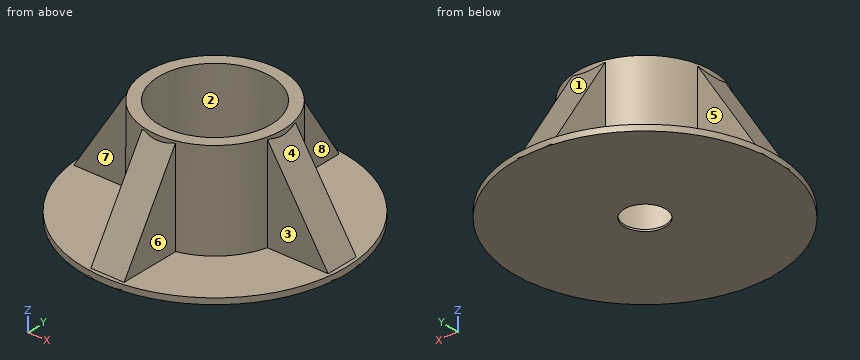
from build123d import *

# Parameters (mm, degrees)
F4_DEPTH        = 7.5
F4_COPIES_COUNT = 4


# Not quite as in the source:
# - a pattern or mirror of a feature is missing from the dataset's text; its kind, count and spacing are read off the source's solid


with BuildPart() as f2:
    # F0 (on Front) → F2 (revolve)
    with BuildSketch(Plane.XZ):
        Polygon((9.3577429652, 0), (59.3534484506, 0), (59.3534484506, 2.7155173011), (30.840517953, 2.7155173011), (30.840517953, 46.9396561384), (25.4094842821, 46.9396561384), (25.7850456983, 0.8370543364), (9.3577429652, 0.8370543364), align=None)
    revolve(axis=Axis((0, 0, 37.2192747891), (0, 0, 1)))

    # F3 (on Front) → F4 (join, symmetric)
    with BuildSketch(Plane.XZ):
        Polygon((59.184409678, 0), (30.097162351, 45.9310486913), (30.097162351, 0), align=None)
    f4 = extrude(amount=F4_DEPTH, both=True)

    # F4_copies: F4 ×4 about axis
    f4_copies_axis = Axis((0, 0, 0), (0, 0, 1))
    for i in range(1, F4_COPIES_COUNT):
        add(f4.rotate(f4_copies_axis, i * 360 / F4_COPIES_COUNT))


solid = f2.part
Verification items for the finished model (mm, model axes). Face numbers are marked on the shaded views. A direction names the side the tool comes from. Round coordinates to 2 decimals unless told otherwise and drop trailing zeros. Loops run counter-clockwise (first coordinate to the right, second up) from the corner with the lowest first, then second, coordinate; pieces in that order, holes last. Notation, with made-up numbers: (83, 69.25) - (102, 69.25) arc R21 cw to (102, 86.25) - close; hole circle Ø5 at (55, -12). An arc over 180 degrees is marked (long way). Answer in a Markdown table with one row per item. Add a question column.
Q1. Section check B-B on x = -43. Enter the section's corners in (y, z), plus the area to 3 significant figures.
Q2. Section check C-C on y = -27.5. Enter the section's corners in (x, z), plus the area to 3 significant figures.
Q3. Section check A-A on z = 4.5. Enter the section's corners in (x, y), plus the area to 3 significant figures.
Q4. Tool access check on the marked faces 5, 6, 7 and 8. Record the directions out of +Z, -Z, +X, -X, +Y, -Y that give a thin tool (end or side, any length) a straight path to the whole face; none if there is none.
Q5. Gauge pin test, flat ends, axial feed: pin 1 (0.6 mm diameter, centred on y = 7, z = 24, fed in from -X); pin 2 (1.5 mm diameter, centred on x = 37, y = 17.5, fed in from +Z); pin 3 (8 mm diameter, centred on x = -27.5, z = 14, fed in from +Y). Record the tip position at first contact, or that the pin passes through.
Q6. Section check D-D on z = 16.5. Enter the section's corners in (x, y).
Q7. Release check for a two-part mould opening along Y. For the marked faces 1, 2, 3 and 4 record: pulls with the +Y half, pulls with the -Y half, needs draft (parallel to the pull), parting line crosses it, or undercut.
Q8. Material ranges on line 1 (Y direction, x = 0, z = 0.25); line 2 (Z direction, x = 23.5, y = 42); line 3 (X direction, y = 33.5, z = 8.5), recorded low to high.
Found:
| question | item | result |
|---|---|---|
| 1 | outline | (-40.91, 0) - (40.91, 0) - (40.91, 2.72) - (7.5, 2.72) - (7.5, 25.56) - (-7.5, 25.56) - (-7.5, 2.72) - (-40.91, 2.72) - close |
| 1 | area | 565 mm² |
| 2 | outline | (-52.6, 0) - (52.6, 0) - (52.6, 2.72) - (13.96, 2.72) - (13.96, 46.94) - (-13.96, 46.94) - (-13.96, 2.72) - (-52.6, 2.72) - close |
| 2 | area | 1,520 mm² |
| 3 | outline | (-56.33, -7.5) - (-30.1, -7.5) - (-30.1, -6.73) arc R30.84 ccw to (-6.73, -30.1) - (-7.5, -30.1) - (-7.5, -56.33) - (7.5, -56.33) - (7.5, -30.1) - (6.73, -30.1) arc R30.84 ccw to (30.1, -6.73) - (30.1, -7.5) - (56.33, -7.5) - (56.33, 7.5) - (30.1, 7.5) - (30.1, 6.73) arc R30.84 ccw to (6.73, 30.1) - (7.5, 30.1) - (7.5, 56.33) - (-7.5, 56.33) - (-7.5, 30.1) - (-6.73, 30.1) arc R30.84 ccw to (-30.1, 6.73) - (-30.1, 7.5) - (-56.33, 7.5) - close; hole circle Ø51.51 at (0, 0) |
| 3 | area | 2,450 mm² |
| 4 | face 5 | +Z, -X, +Y |
| 4 | face 6 | +Z, +X, -Y |
| 4 | face 7 | +Z, -X, -Y |
| 4 | face 8 | +Z, +X, +Y |
| 5 | pin 1 | stops at x = -44.18 |
| 5 | pin 2 | stops at z = 2.72 |
| 5 | pin 3 | stops at y = 19.97 |
| 6 | outline | (-48.74, -7.5) - (-30.1, -7.5) - (-30.1, -6.73) arc R30.84 ccw to (-6.73, -30.1) - (-7.5, -30.1) - (-7.5, -48.74) - (7.5, -48.74) - (7.5, -30.1) - (6.73, -30.1) arc R30.84 ccw to (30.1, -6.73) - (30.1, -7.5) - (48.74, -7.5) - (48.74, 7.5) - (30.1, 7.5) - (30.1, 6.73) arc R30.84 ccw to (6.73, 30.1) - (7.5, 30.1) - (7.5, 48.74) - (-7.5, 48.74) - (-7.5, 30.1) - (-6.73, 30.1) arc R30.84 ccw to (-30.1, 6.73) - (-30.1, 7.5) - (-48.74, 7.5) - close; hole circle Ø51.31 at (0, 0) |
| 7 | face 1 | pulls with the +Y half |
| 7 | face 2 | undercut |
| 7 | face 3 | pulls with the -Y half |
| 7 | face 4 | needs draft |
| 8 | line 1 | y = -59.35 to -9.36, 9.36 to 59.35 |
| 8 | line 2 | z = 0 to 2.72 |
| 8 | line 3 | x = -7.5 to 7.5 |
